The listing builds one solid part. Answer for the finished solid, in the listing's coordinates (mm). Face numbers are marked on the shaded views. A direction names the side the tool comes from. Coordinates: 2 decimals unless noted, no trailing zeros. Loops run counter-clockwise (first coordinate to the right, second up) from the corner with the lowest first, then second, coordinate; pieces in that order, holes last. Notation, with made-up numbers: (-18, 23) - (34, 23) arc R20 ccw to (34, 61) - close; hole circle Ø8 at (26.25, 63.25). An arc over 180 degrees is marked (long way). Use one line per item in the form item = value. Start each with the question number.
```python
from build123d import *

# Parameters (mm, degrees)
F0_W     = 101.6
F0_H     = 101.6
F1_DEPTH = 101.6
F2_W     = 101.6
F2_H     = 82.4549061418
F3_DEPTH = 76.2
F4_W     = 50.8
F4_H     = 25.4
F5_DEPTH = 50.546
F6_W     = 50.8
F6_H     = 19.1450938582
F7_DEPTH = 50.8
F9_DEPTH = 136.906


with BuildPart() as f1:
    # F0 (on Front) → F1 (new body)
    with BuildSketch(Plane.XZ):
        with Locations((-50.8, -50.8)):
            Rectangle(F0_W, F0_H)
    extrude(amount=F1_DEPTH)

    # F2 (on face) → F3 (cut)
    with BuildSketch(Plane.XY):
        with Locations((-50.8, -60.3725469291)):
            Rectangle(F2_W, F2_H)
    extrude(amount=-F3_DEPTH, mode=Mode.SUBTRACT)

    # F4 (on face) → F5 (cut)
    with BuildSketch(Plane.XY.offset(-76.2)):
        with Locations((-50.8, -88.9)):
            Rectangle(F4_W, F4_H)
    extrude(amount=-F5_DEPTH, mode=Mode.SUBTRACT)

    # F6 (on face) → F7 (cut)
    with BuildSketch(Plane.XY):
        with Locations((-50.8, -9.5725469291)):
            Rectangle(F6_W, F6_H)
    extrude(amount=-F7_DEPTH, mode=Mode.SUBTRACT)

    # F8 (on face) → F9 (cut)
    with BuildSketch(Plane.XZ.offset(19.1450938582)):
        Polygon((-101.6, 0), (-101.6, -25.4), (-76.2, 0), align=None)
        Polygon((-25.4, 0), (0, -25.4), (0, 0), align=None)
    extrude(amount=-F9_DEPTH, mode=Mode.SUBTRACT)


solid = f1.part
```
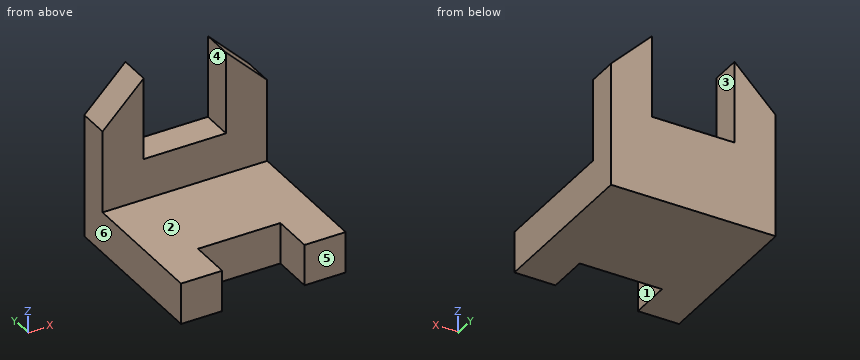
(1) Each of these flat-tipped pins is pushed along its axis until it touches: pin 1 Ø7.5 at (x, z) = (-43.5, -95) entering from -Y; pin 2 Ø1.5 at (x, y) = (-62.5, -18.5) entering from +Z; pin 3 Ø10 at (x, y) = (-13.5, -10.5) entering from +Z. Where does it stop, or does it pass through?
(2) For the marked faces 1, 2 and 3, determine the directions among +Z, -Z, +X, -X, +Y, -Y from which every point of the face is accessible in a straight line to the end or side of a thin tool.
(3) Find the intervals of material crossed by probe 1 along Z at (x, y) = (-15.5, -85.5); probe 2 along Y at (x, z) = (-87.5, -43.5); probe 3 along X at (y, z) = (-85, -89), in increasing order. Write a range as from..to.
(4) Determine the mould class of the marked faces 4, 5 and 6 for opening direction X: +X half, -X half, draft (parallel to the pull), parting line (faces both ways), or undercut.
(5) A cutting plane is placed at D-D (z = -89). Determine the outline of the cut face in (x, y).
(6) A cutting plane is placed at B-B (y = -88). Determine the outline of the cut face in (x, z), then the cut area to 3 significant figures.
(7) A cutting plane is placed at C-C (y = -10). Determine the outline of the cut face in (x, z), then the cut area to 3 significant figures.
(8) A cutting plane is placed at A-A (z = -22). Determine the outline of the cut face in (x, y), then the cut area to 3 significant figures.
Evaluation:
q1.pin_1 = -76.2
q1.pin_2 = -50.8
q1.pin_3 = -6.9
q2.face_1 = +Z, -Z, -Y
q2.face_2 = +Z, +X, -X, -Y
q2.face_3 = +Z, +Y, -Y
q3.probe_1 = -101.6..-76.2
q3.probe_2 = -19.15..0
q3.probe_3 = -101.6..-76.2, -25.4..0
q4.face_4 = undercut
q4.face_5 = draft
q4.face_6 = -X half
q5.outline = (-101.6, -101.6) - (-76.2, -101.6) - (-76.2, -76.2) - (-25.4, -76.2) - (-25.4, -101.6) - (0, -101.6) - (0, 0) - (-101.6, 0) - close
q6.outline = (-101.6, -101.6) - (-76.2, -101.6) - (-76.2, -76.2) - (-101.6, -76.2) - close; (-25.4, -101.6) - (0, -101.6) - (0, -76.2) - (-25.4, -76.2) - close
q6.area = 1,290 mm^2
q7.outline = (-101.6, -101.6) - (0, -101.6) - (0, -25.4) - (-25.4, 0) - (-25.4, -50.8) - (-76.2, -50.8) - (-76.2, 0) - (-101.6, -25.4) - close
q7.area = 7,100 mm^2
q8.outline = (-98.2, -19.15) - (-76.2, -19.15) - (-76.2, 0) - (-98.2, 0) - close; (-25.4, -19.15) - (-3.4, -19.15) - (-3.4, 0) - (-25.4, 0) - close
q8.area = 842 mm^2
